Source: CAD feature listing. Evaluate the final solid. Frame: model axes, mm. A direction names the side the tool comes from. Give positions to 0.01 mm unless a question says otherwise; leave off trailing zeros. Loops run counter-clockwise (first coordinate to the right, second up) from the corner with the lowest first, then second, coordinate; pieces in that order, holes last. Notation, with made-up numbers: M 3,14.5 L 11,14.5 A18 cw 11,20.5 Z; hole C 43,14.5 d1. An arc over 180 degrees is marked long. Answer in a Markdown table with one row per item.
```python
from build123d import *

# Parameters (mm, degrees)
SKETCH1_W           = 40
SKETCH1_H           = 40
BOSS_EXTRUDE1_DEPTH = 40
CUT_EXTRUDE1_DEPTH  = 20
CUT_EXTRUDE2_DEPTH  = 60
CUT_EXTRUDE3_DEPTH  = 60


with BuildPart() as part:
    # Sketch1 → Boss-Extrude1 (new body)
    with BuildSketch(Plane(origin=(0, 0, 0), x_dir=(0, 0, -1), z_dir=(1, 0, 0))):
        with Locations((20, 20)):
            Rectangle(SKETCH1_W, SKETCH1_H)
    extrude(amount=BOSS_EXTRUDE1_DEPTH)

    # Sketch2 → Cut-Extrude1 (cut)
    with BuildSketch(Plane(origin=(40, 0, 0), x_dir=(0, 0, -1), z_dir=(1, 0, 0))):
        Polygon((0, 0), (40, 40), (40, 0), align=None)
    extrude(amount=-CUT_EXTRUDE1_DEPTH, mode=Mode.SUBTRACT)

    # Sketch3 → Cut-Extrude2 (cut)
    with BuildSketch(Plane.XY):
        Polygon((0, 0), (20, 0), (0, 40), align=None)
        Polygon((40, 40), (20, 0), (40, 0), align=None)
    extrude(amount=-CUT_EXTRUDE2_DEPTH, mode=Mode.SUBTRACT)

    # Sketch4 → Cut-Extrude3 (cut)
    with BuildSketch(Plane(origin=(0, 0, 0), x_dir=(1, 0, 0), z_dir=(0, 1, 0))):
        Polygon((0, 0), (20, 0), (0, 40), align=None)
        Polygon((40, 40), (20, 0), (40, 0), align=None)
    extrude(amount=CUT_EXTRUDE3_DEPTH, mode=Mode.SUBTRACT)


solid = part.part
```
1) Section A-A, the plane y = 5. Return loops of the section in (x, z).
Reply:
| item | result |
|---|---|
| outline | M 17.5,-40 L 20,-40 L 20,-5 L 22.5,-5 L 20,0 L 17.5,-5 Z |
2) Pin query (flat end, axial travel): pin 1 Ø1 at (x, z) = (32, -27) entering from -Y; pin 2 Ø10 at (x, y) = (25.5, 29.5) entering from -Z; pin 3 Ø2 at (x, z) = (18.5, -29) entering from -Y. Return the tip coordinate at first contact, or that it passes through.
Reply:
| item | result |
|---|---|
| pin 1 | stops at y = 26.5 |
| pin 2 | stops at z = -34.5 |
| pin 3 | stops at y = 1 |
3) Set-up query: faces 1 (the flat face through (26, 29, -29)), 2 (the flat face through (25.7, 28.6, -11.4)). Return all of +Z, -Z, +X, -X, +Y, -Y with unobstructed straight access to the full face (end or side cutting, diameter ignored); none if empty.
Reply:
| item | result |
|---|---|
| face 1 | -Z, +X, -Y |
| face 2 | +Z, +X, +Y, -Y |
4) Section B-B, the plane z = -3. Return loops of the section in (x, y), then the cut area to 3 significant figures.
Reply:
| item | result |
|---|---|
| outline | M 18.5,3 L 20,0 L 20,3 L 21.5,3 L 21.5,40 L 18.5,40 Z |
| area | 113 mm² |
5) Section C-C, the plane x = 37. Return loops of the section in (y, z), then the cut area to 3 significant figures.
Reply:
| item | result |
|---|---|
| outline | M 34,-34 L 40,-40 L 40,-34 Z |
| area | 18.0 mm² |
6) Material intervals for L1, parallel to Y at x = 16.5, z = -35.5; L2, parallel to Y at x = 11, z = -37; L3, parallel to Z at x = 9, y = 32, sorted ascending.
Reply:
| item | result |
|---|---|
| L1 | y = 7 to 40 |
| L2 | y = 18 to 40 |
| L3 | z = -40 to -22 |
7) Section D-D, the plane x = 4. Return loops of the section in (y, z).
Reply:
| item | result |
|---|---|
| outline | M 32,-40 L 40,-40 L 40,-32 L 32,-32 Z |
